```python
from build123d import *

# Parameters (mm, degrees)
F1_DEPTH = 6
F4_R     = 0.7


with BuildPart() as f1:
    # F0 (on Top) → F1 (new body)
    with BuildSketch(Plane.XY):
        Polygon((7.05, -4.0703193978), (7.05, 4.0703193978), (0, 8.1406387956), (-7.05, 4.0703193978), (-7.05, -4.0703193978), (0, -8.1406387956), align=None)
    extrude(amount=F1_DEPTH)

    # F2 (on Right) → F3 (revolve, cut)
    with BuildSketch(Plane.YZ):
        with BuildLine():
            Line((0, -10), (0, 0))
            Line((0, 0), (0, 1))
            ThreePointArc((0, 1), (-11, -10), (0, -21))
            Line((0, -21), (0, -10))
        make_face()
    revolve(axis=Axis((0, 0, -5), (0, 0, -1)), mode=Mode.SUBTRACT)

    # F4
    f4_edges = [f1.edges().sort_by_distance(p)[0] for p in [
        (3.525, -6.105479, 6),
        (7.05, 0, 6),
        (3.525, 6.105479, 6),
        (-3.525, 6.105479, 6),
        (-7.05, 0, 6),
        (-3.525, -6.105479, 6),
        (3.525, -6.105479, 0),
        (-3.525, -6.105479, 0),
        (7.05, 0, 0),
        (-7.05, 0, 0),
        (3.525, 6.105479, 0),
        (-3.525, 6.105479, 0),
        (0, 4.582576, 0),
    ]]
    fillet(f4_edges, radius=F4_R)


solid = f1.part
```
Check sheet for the modelled part. Datum: model origin and axes. Units: mm. Give positions to 0.01 mm unless a question says otherwise; leave off trailing zeros. Write each loop counter-clockwise with the first axis right and the second up, starting at its lowest first coordinate (ties: lowest second). Pieces come first, ordered by that corner, then holes.
Item 1: Cross-section at A-A (z = 3.75). Enter the section's corners in (x, y), and give its area (3 significant figures).
Item 2: Cross-section at B-B (z = 5.5). Enter the section's corners in (x, y).
Item 3: Scan lines: L1, parallel to X at y = -5.25, z = 5.25; L2, parallel to Z at x = -1, y = -7.5; L3, parallel to Z at x = 3.75, y = 0.75. Record each from-to range of solid material in increasing order.
Item 4: Gauge pin test, flat end, axial feed: pin 1 (5 mm diameter, centred on x = -2.5, y = -1, fed in from -Z). Record the tip position at first contact, or that the pin passes through.
Report:
1. outline: (-7.05, -4.07) - (0, -8.14) - (7.05, -4.07) - (7.05, 4.07) - (0, 8.14) - (-7.05, 4.07) - close
1. area: 172 mm2
2. outline: (-7.02, -4.05) - (0, -8.11) - (7.02, -4.05) - (7.02, 4.05) - (0, 8.11) - (-7.02, 4.05) - close
3. L1: x = -5.01 to 5.01
3. L2: z = 0.43 to 5.57
3. L3: z = 0.31 to 6
4. pin 1: stops at z = 0
